Check sheet for the drawn part. Datum: minimum x, y, z corner. Units: mm. A direction names the side the tool comes from. Give positions to 0.01 mm unless a question says otherwise; leave off trailing zeros. Write each loop counter-clockwise with the first axis right and the second up, starting at its lowest first coordinate (ties: lowest second). Pieces come first, ordered by that corner, then holes. Notation, with made-up numbers: (49, 16) -> (72, 16) arc R16 ccw to (72, 30) -> close; hole circle Ø2 at (77, 61). An arc over 180 degrees is marked (long way). Write item = value, one per line. Start each with the question number.
1. Thickness scan on line 1 along Y through (x, z) = (0.6, 6); line 2 along X through (y, z) = (0.7, 6); line 3 along Y through (x, z) = (5.5, 4.5). Record the ranges inside material, lowest first.
2. Cross-section at C-C, the plane x = 12.25. Record the cut outline in (y, z).
3. Cross-section at D-D, the plane z = 10. Record the cut outline in (x, y), plus the area to 3 significant figures.
4. Cross-section at A-A, the plane z = 6. Record the cut outline in (x, y).
5. Cross-section at B-B, the plane y = 12. Record the cut outline in (x, z), plus the area to 3 significant figures.
6. Depth check by flat-ended pin: P1, Ø6, axis at x = 4.5, z = 4.5, coming from the +Y side; P2, Ø2, axis at x = 10.5, z = 7.5, coming from the +Y side; P3, Ø2, axis at y = 8, z = 1.5, coming from the +X side; P4, Ø4.5, axis at x = 13, z = 6, coming from the -Y side. Enter the tip coordinate at first touch or a pass-through.
7. Set-up check for the marked faces 4 and 5: record each of +Z, -Z, +X, -X, +Y, -Y from which the full face is reachable in a straight line by a thin tool's end or side.
8. Mould release check, pull along Z, two halves, no side actions. Record for the marked faces 1, 2 and 3: pulls with the +Z half, pulls with the -Z half, needs draft (parallel to the pull), parting line crosses it, or undercut.
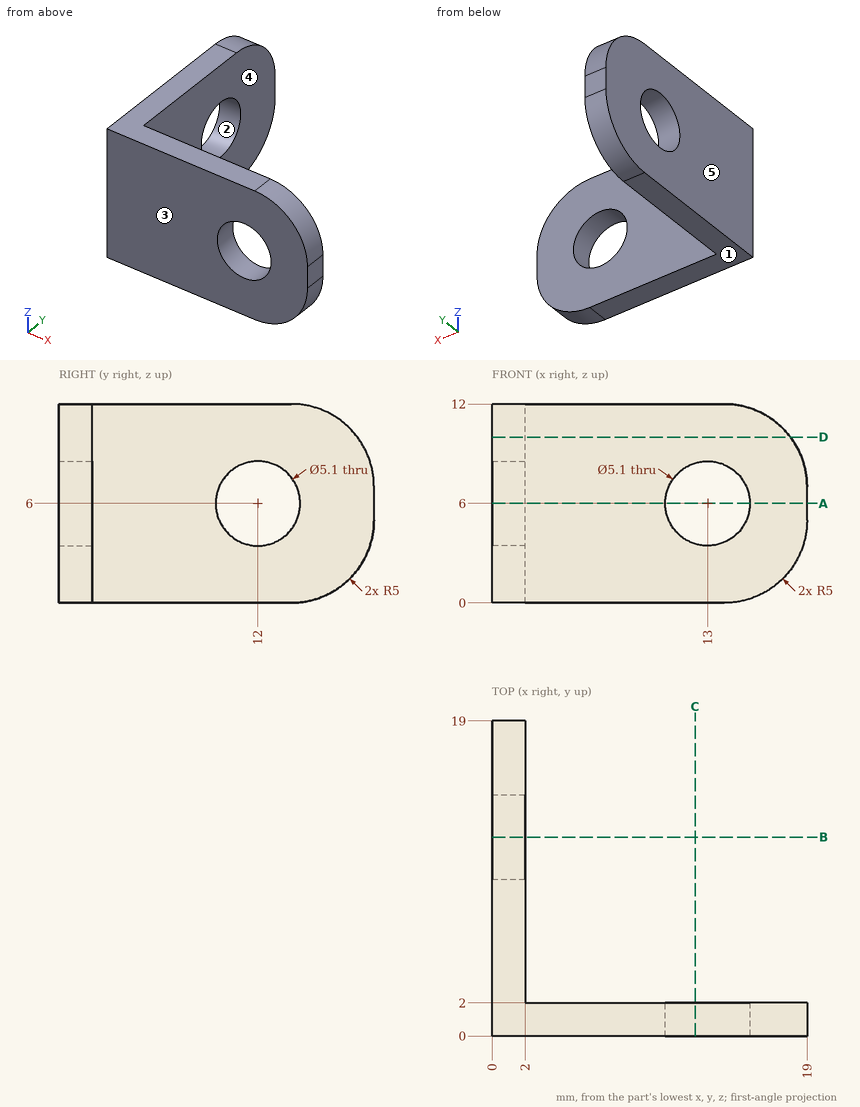
Answers:
q1.line_1 = 0 to 9.45, 14.55 to 19
q1.line_2 = 0 to 10.45, 15.55 to 19
q1.line_3 = 0 to 2
q2.outline = (0, 0) -> (2, 0) -> (2, 3.56) -> (0, 3.56) -> close; (0, 8.44) -> (2, 8.44) -> (2, 12) -> (0, 12) -> close
q3.outline = (0, 0) -> (18, 0) -> (18, 2) -> (2, 2) -> (2, 18) -> (0, 18) -> close
q3.area = 68.0 mm^2
q4.outline = (0, 0) -> (10.45, 0) -> (10.45, 2) -> (2, 2) -> (2, 9.45) -> (0, 9.45) -> close; (0, 14.55) -> (2, 14.55) -> (2, 19) -> (0, 19) -> close; (15.55, 0) -> (19, 0) -> (19, 2) -> (15.55, 2) -> close
q5.outline = (0, 0) -> (2, 0) -> (2, 3.45) -> (0, 3.45) -> close; (0, 8.55) -> (2, 8.55) -> (2, 12) -> (0, 12) -> close
q5.area = 13.8 mm^2
q6.P1 = 19
q6.P2 = 2
q6.P3 = 2
q6.P4 = through
q7.face_4 = +Z, -Z, +X, +Y
q7.face_5 = +Z, -Z, -X, +Y, -Y
q8.face_1 = pulls with the -Z half
q8.face_2 = undercut
q8.face_3 = needs draft
